from build123d import *

# Parameters (mm, degrees)
F0_R     = 2.8
F1_DEPTH = 2.6
F2_R     = 2.8
F3_DEPTH = 2.6
F4_R     = 3
F5_R     = 1


with BuildPart() as f1:
    # F0 (on Top) → F1 (new body)
    with BuildSketch(Plane.XY):
        with BuildLine():
            Line((0, 18.5), (0, 0))
            Line((0, 0), (64, 0))
            Line((64, 0), (64, 12.9))
            ThreePointArc((64, 12.9), (62.3597979746, 16.8597979746), (58.4, 18.5))
            Line((58.4, 18.5), (0, 18.5))
        make_face()
        with Locations((7.4, 11.1)):
            Circle(F0_R, mode=Mode.SUBTRACT)
        with Locations((56.6, 11.1)):
            Circle(F0_R, mode=Mode.SUBTRACT)
    extrude(amount=F1_DEPTH)

    # F2 (on Front) → F3 (join)
    with BuildSketch(Plane.XZ):
        with BuildLine():
            Line((0, 19.8681156561), (0, 1.3681156561))
            Line((0, 1.3681156561), (64, 1.3681156561))
            Line((64, 1.3681156561), (64, 14.2681156561))
            ThreePointArc((64, 14.2681156561), (62.3597979746, 18.2279136307), (58.4, 19.8681156561))
            Line((58.4, 19.8681156561), (0, 19.8681156561))
        make_face()
        with Locations((7.4, 12.4681156561)):
            Circle(F2_R, mode=Mode.SUBTRACT)
        with Locations((56.6, 12.4681156561)):
            Circle(F2_R, mode=Mode.SUBTRACT)
    extrude(amount=-F3_DEPTH)

    # F4
    f4_edges = [f1.edges().sort_by_distance(p)[0] for p in [
        (32, 0, 0),
        (32, 2.6, 2.6),
    ]]
    fillet(f4_edges, radius=F4_R)

    # F5
    f5_edges = [f1.edges().sort_by_distance(p)[0] for p in [
        (29.2, 2.6, 19.868116),
        (29.2, 0, 19.868116),
        (29.2, 18.5, 2.6),
        (29.2, 18.5, 0),
        (64, 0, 8.634058),
        (64, 0.87868, 0.87868),
        (64, 7.95, 0),
        (64, 9.25, 2.6),
        (64, 2.6, 9.934058),
        (62.359798, 2.6, 18.227914),
        (62.359798, 0, 18.227914),
        (62.359798, 16.859798, 2.6),
        (62.359798, 16.859798, 0),
    ]]
    fillet(f5_edges, radius=F5_R)


solid = f1.part
Here's how the part is built. I have some questions about the finished solid (model axes, mm). A direction names the side the tool comes from. Coordinates: 2 decimals unless noted, no trailing zeros. Order: outer loops, then holes, each group sorted by start corner. A loop starts at its lowest first (then second) coordinate and runs counter-clockwise, first axis right, second up. Notation, with made-up numbers: M 84.5,-18.5 L 128.5,-18.5 A14 cw 128.5,-5.5 Z; hole C -6,-34.75 d5. An arc over 180 degrees is marked long. Answer as CSV lines item,"result". Start each with the question number.
1. For pin 1 (10.5 mm diameter, centred on x = 18, z = 10.5, fed in from +Y); pin 2 (5 mm diameter, centred on x = 56.6, y = 11.1, fed in from -Z); pin 3 (6 mm diameter, centred on x = 31.5, y = 14, fed in from +Z), each with a flat end and sliding along its axis, tell me the tip position at first contact or that it passes through.
2. I want a section at D-D, the plane z = 11. Write out the boundary of the cut face in (x, y).
3. I want a section at B-B, the plane y = 9.25. Write out the boundary of the cut face in (x, z).
4. We'd pull the mould along Y, two halves only. Please class faces 3 (the cylindrical face through (4.6, 11.2, 1.3)), 4 (the flat face through (31, 0, 11)), 5 (the cylindrical face through (53.8, 11.2, 1.3)), 6 (the flat face through (31, 10, 0)): released by +Y, released by -Y, zero draft, split by the parting line, or undercut.
5. I want a section at C-C, the plane x = 49. Write out the boundary of the cut face in (y, z), and give its area (3 significant figures).
6. I want a section at A-A, the plane x = 7.4. Write out the boundary of the cut face in (y, z), and give its area (3 significant figures).
7. On a 3-axis mill with a long thin cutter (end or side, diameter ignored), from which of +Z, -Z, +X, -X, +Y, -Y can I reach the whole of each face in a straight line? I mean faces 1 (the flat face through (31, 12, 2.6)), 2 (the cylindrical face through (54.536, 1.282, 14.36)). Say none if no direction works.
8. I need wall thicknesses on line 1 (Z direction, x = 26, y = 15.5); line 2 (Y direction, x = 7.4, z = 2). Which ranges of each line are inside material? Lowest first, please. Write a range as [from, to].
Recorded:
1,pin 1,"stops at y = 2.62"
1,pin 2,"passes through"
1,pin 3,"stops at z = 2.6"
2,outline,"M 0,0 L 5.02,0 L 5.02,2.6 L 0,2.6 Z; M 9.78,0 L 54.22,0 L 54.22,2.6 L 9.78,2.6 Z; M 58.98,0 L 63,0 A1 ccw 64,1 L 64,1.6 A1 ccw 63,2.6 L 58.98,2.6 Z"
3,outline,"M 0,0 L 5.3,0 L 5.3,2.6 L 0,2.6 Z; M 9.5,0 L 54.5,0 L 54.5,2.6 L 9.5,2.6 Z; M 58.7,0 L 63,0 A1 ccw 64,1 L 64,1.6 A1 ccw 63,2.6 L 58.7,2.6 Z"
4,face 3,"undercut"
4,face 4,"released by -Y"
4,face 5,"undercut"
4,face 6,"zero draft"
5,outline,"M 0,3 A3 ccw 3,0 L 17.5,0 A1 ccw 18.5,1 L 18.5,1.6 A1 ccw 17.5,2.6 L 5.6,2.6 A3 cw 2.6,5.6 L 2.6,18.87 A1 ccw 1.6,19.87 L 1,19.87 A1 ccw 0,18.87 Z"
5,area,"92.1 mm2"
6,outline,"M 0,3 A3 ccw 3,0 L 8.3,0 L 8.3,2.6 L 5.6,2.6 A3 cw 2.6,5.6 L 2.6,9.67 L 0,9.67 Z; M 0,15.27 L 2.6,15.27 L 2.6,18.87 A1 ccw 1.6,19.87 L 1,19.87 A1 ccw 0,18.87 Z; M 13.9,0 L 17.5,0 A1 ccw 18.5,1 L 18.5,1.6 A1 ccw 17.5,2.6 L 13.9,2.6 Z"
6,area,"63.0 mm2"
7,face 1,"+Z, +X, -X, +Y"
7,face 2,"+Y, -Y"
8,line 1,"z = [0, 2.6]"
8,line 2,"y = [0.17, 8.3], [13.9, 18.42]"
